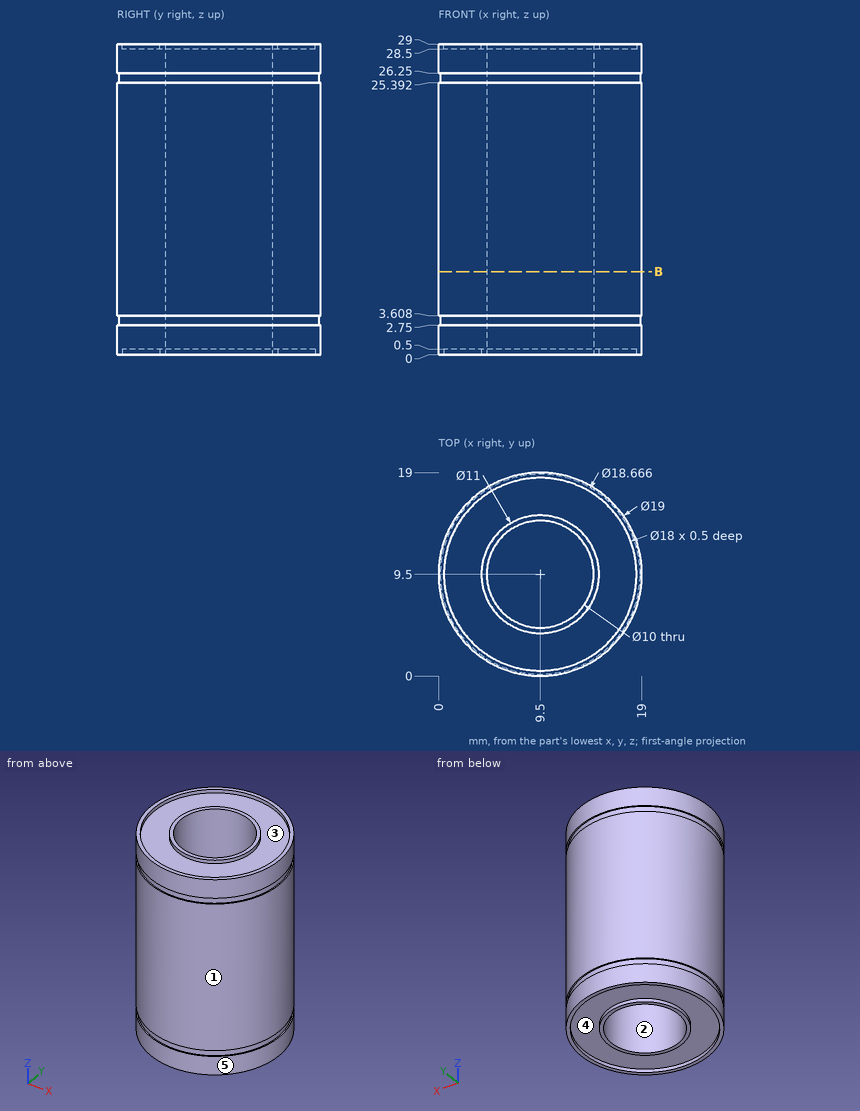
Geometry check sheet. Reference: drawing and pictorial views, mm from the part's lowest x, y, z. A direction names the side the tool comes from. Coordinates: 2 decimals unless noted, no trailing zeros. Write each loop counter-clockwise with the first axis right and the second up, starting at its lowest first coordinate (ties: lowest second). Pieces come first, ordered by that corner, then holes. Notation, with made-up numbers: (-37.75, 45.5) -> (-17.75, 45.5) arc R23 ccw to (-17.75, 75.5) -> close; hole circle Ø3 at (65, 13). An arc over 180 degrees is marked (long way). One line per question, with ' | ' between items.
1. Draft check along X on the marked faces 1 and 2. Enter one of: +X half, -X half, draft (parallel to the pull), parting line (faces both ways), or undercut.
Answers:
face 1: parting line | face 2: undercut
2. Thickness scan on probe 1 along Y at (x, z) = (9.5, 28.7); probe 2 along Y at (x, z) = (5, 12) (1 decimal); probe 3 along X at (y, z) = (11.5, 4). Record the ranges inside material, lowest first. Write a range as from..to.
Answers:
probe 1: y = 0..0.5, 4..4.5, 14.5..15, 18.5..19 | probe 2: y = 1.1..7.3, 11.7..17.9 | probe 3: x = 0.21..4.92, 14.08..18.79
3. Cross-section at B-B on z = 7.75. Record the cut outline in (x, y).
Answers:
outline: circle Ø19 at (9.5, 9.5); hole circle Ø10 at (9.5, 9.5)
4. Set-up check for the marked faces 3, 4 and 5: record each of +Z, -Z, +X, -X, +Y, -Y from which the full face is reachable in a straight line by a thin tool's end or side.
Answers:
face 3: +Z | face 4: -Z | face 5: +Z, -Z
5. Depth check by flat-ended pin: pin 1 Ø6 at (x, y) = (16.5, 16.5) entering from +Z; pin 2 Ø10 at (y, z) = (2, 15) entering from +X (1 decimal); pin 3 Ø5 at (x, z) = (2.5, 12) entering from +Y; pin 4 Ø10 at (y, z) = (15.5, 3) entering from +X. Enter the tip coordinate at first touch or a pass-through.
Answers:
pin 1: stops at z = 29 | pin 2: stops at x = 18.7 | pin 3: stops at y = 17.87 | pin 4: stops at x = 18.95
